For this review, take the finished solid that the model builds, in its own axes (mm). Coordinates: 2 decimals unless noted, no trailing zeros. Order: outer loops, then holes, each group sorted by start corner. A loop starts at its lowest first (then second) coordinate and runs counter-clockwise, first axis right, second up. Notation, with made-up numbers: (28.5, -18) -> (36.5, -18) arc R28 ccw to (36.5, 11) -> close; hole circle Ø1 at (64, -14.5). An arc over 180 degrees is marked (long way). Write item = value, one per line. Start each with the question number.
1) Insertion check: pin 1 Ø3.5 at (y, z) = (70.5, -201) entering from +X; pin 2 Ø6 at (x, z) = (186, -169.5) entering from +Y; pin 3 Ø13 at (y, z) = (65, -202.5) entering from -X. Each pin has a flat end and moves straight along its axis. Give the tip position at first contact, or say it passes through.
2) Consider section A-A on x = 330. Give the boundary of the cut face in (y, z).
3) Consider section B-B on y = 68. Give the boundary of the cut face in (x, z), and give its area (3 significant figures).
4) Wall thickness on probe 1 along Y at (x, z) = (370, -141.5): over which ranges is the line inside the solid? List them lowest first. Write a range as [from, to].
5) Consider section C-C on x = 257. Give the boundary of the cut face in (y, z).
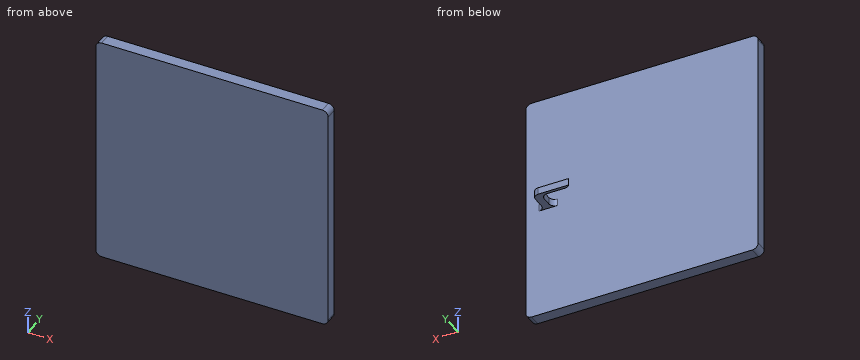
Autodesk Inventor part; units mm, degrees
ref_plane "YZ Plane" through (0, 0, 0) normal (1, 0, 0) x (0, 1, 0)
ref_plane "XZ Plane" through (0, 0, 0) normal (0, 1, 0) x (-1, 0, 0)
ref_plane "XY Plane" through (0, 0, 0) normal (0, 0, 1) x (1, 0, 0)
sketch "Sketch1" plane through (0, 0, 0) normal (0, 1, 0) x (-1, 0, 0)
  point P0 (0, 0)
sketch "Sketch2" plane through (0, 0, 0) normal (0, 1, 0) x (-1, 0, 0)
  line L0 (0, 0) -> (-400, 0)
  line L1 (-400, 0) -> (-400, -400)
  line L2 (-400, -400) -> (0, -400)
  line L3 (0, -400) -> (0, 0)
  dimension "d0" = 400
  dimension "d1" = 400
extrude "Extrusion1" add sketch "Sketch2" along normal blind 50
sketch "Sketch3" plane through (0, 50, 0) normal (0, 1, 0) x (1, 0, 0)
  line L0 (0, 400) -> (0, 0)
  line L1 (0, 200) -> (400, 200)
  line L2 (400, 0) -> (400, 400)
  line L3 (330.1231, 200) -> (330.1231, 206)
  line L4 (330.1231, 200) -> (330.1231, 194)
  line L5 (330.1231, 194) -> (325.1231, 194)
  line L6 (325.1231, 194) -> (325.1231, 206)
  line L7 (325.1231, 206) -> (330.1231, 206)
  dimension "d4" = 6
  dimension "d5" = 6
  dimension "d6" = 5
extrude "Extrusion2" add sketch "Sketch3" along normal blind 40
sketch "Sketch4" plane through (0, 0, 0) normal (0, -1, 0) x (1, 0, 0)
  line L0 (400, -400) -> (0, -400)
  line L1 (400, 0) -> (400, -400)
  line L2 (0, -400) -> (400, -400)
  line L3 (400, -400) -> (400, 0)
  line L4 (400, 0) -> (0, 0)
  line L5 (0, 0) -> (0, -400)
extrude "Extrusion3" cut sketch "Sketch4" against normal blind 30
fillet "Fillet1" radius 10 4 edges at (0, 40, 0) (0, 40, -400) (400, 40, -400) (400, 40, 0)
sketch "Sketch5" plane through (330.1231, 50, -194) normal (1, 0, 0) x (0, 0, -1)
  line L0 (0, 0) -> (0, 40)
  line L1 (0, 0) -> (12, 0)
  line L2 (0, 40) -> (12, 40)
  line L3 (12, 40) -> (12, 0)
  line L4 (12, 0) -> (0, 0)
  line L5 (0, 0) -> (0, 40)
  point P0 (-194, -50)
extrude "Extrusion4" add sketch "Sketch5" along normal blind 60
sketch "Sketch7" plane through (325.1231, 50, -206) normal (-1, 0, 0) x (0, 0, 1)
  line L0 (0, 40) -> (12, 40)
  line L1 (12, 0) -> (0, 0)
  line L2 (0, 40) -> (12, 40)
  line L3 (12, 40) -> (12, 0)
  line L4 (12, 0) -> (0, 0)
  line L5 (0, 0) -> (0, 40)
  point P0 (206, -50)
extrude "Extrusion6" cut sketch "Sketch7" against normal blind 45
sketch "Sketch8" plane through (390.1231, 50, -194) normal (1, 0, 0) x (0, 0, -1)
  line L0 (12, 40) -> (0, 40)
  line L1 (12, 0) -> (0, 0)
  line L2 (0, 40) -> (12, 40)
  line L3 (12, 40) -> (12, 0)
  line L4 (12, 0) -> (0, 0)
  line L5 (0, 0) -> (0, 40)
  point P0 (-194, -50)
extrude "Extrusion7" add sketch "Sketch8" against normal blind 35
sketch "Sketch9" plane through (390.1231, 50, -194) normal (1, 0, 0) x (0, 0, -1)
  line L0 (12, 40) -> (0, 40)
  line L1 (12, 0) -> (12, 40)
  line L2 (0, 40) -> (12, 40)
  line L3 (12, 40) -> (12, 0)
  line L4 (12, 0) -> (0, 0)
  line L5 (0, 0) -> (0, 40)
  point P0 (-194, -50)
extrude "Extrusion8" cut sketch "Sketch9" against normal blind 22.5
sketch "Sketch10" plane through (355.1231, 50, -194) normal (-1, 0, 0) x (0, 0, 1)
  line L0 (-12, 40) -> (-12, 0)
  line L1 (0, 0) -> (0, 40)
  line L2 (-12, 40) -> (0, 40)
  line L3 (0, 40) -> (0, 35)
  line L4 (0, 35) -> (-12, 35)
  line L5 (-12, 35) -> (-12, 40)
  point P0 (194, -50)
  dimension "d22" = 5
extrude "Extrusion9" add sketch "Sketch10" along normal blind 50
fillet "Fillet2" radius 10 5 edges at (367.6231, 90, -200) (355.1231, 85, -200) (305.1231, 85, -200) (355.1231, 50, -200) (367.6231, 50, -200)
sketch "Sketch6" plane through (325.1231, 50, -206) normal (-1, 0, 0) x (0, 0, 1)
  line L0 (0, 0) -> (0, 40)
  line L1 (12, 40) -> (12, 0)
  line L2 (0, 40) -> (12, 40)
  line L3 (12, 40) -> (12, 0)
  line L4 (12, 0) -> (0, 0)
  line L5 (0, 0) -> (0, 40)
  point P0 (206, -50)
properties part number "wood part 2"
Answer sheet:
q1.pin_1 = 367.62
q1.pin_2 = 50
q1.pin_3 = 355.01
q2.outline = (30, -400) -> (50, -400) -> (50, 0) -> (30, 0) -> close; (85, -206) -> (90, -206) -> (90, -194) -> (85, -194) -> close
q3.outline = (355.12, -206) -> (367.62, -206) -> (367.62, -194) -> (355.12, -194) -> close
q3.area = 150 mm2
q4.probe_1 = [30, 50]
q5.outline = (30, -400) -> (50, -400) -> (50, 0) -> (30, 0) -> close
